from build123d import *

# Parameters (mm, degrees)
SKETCH3_R          = 4.141637382
CUT_EXTRUDE1_DEPTH = 7
FILLET2_R          = 1
FILLET3_R          = 1


with BuildPart() as part:
    # Sketch2 → Revolve1 (revolve)
    with BuildSketch(Plane.XY, mode=Mode.PRIVATE) as revolve1_sk:
        with BuildLine():
            Line((1.5, 1.5), (1.5, 3.5))
            ThreePointArc((1.5, 3.5), (1.207106781, 4.207106781), (0.5, 4.5))
            Line((0.5, 4.5), (-9.5, 4.5))
            Line((-9.5, 4.5), (-9.5, 11.5))
            Line((-9.5, 11.5), (9, 11.5))
            Line((9, 11.5), (9, 1.5))
            Line((9, 1.5), (1.5, 1.5))
        make_face()
    revolve(revolve1_sk.sketch.rotate(Axis((9, 1.5, 0), (0, 1, 0)), 270), axis=Axis((9, 1.5, 0), (0, 1, 0)))

    # Sketch3 → Cut-Extrude1 (cut)
    with BuildSketch(Plane.XZ.offset(-1.5)):
        with Locations((9, 0)):
            Circle(SKETCH3_R)
    extrude(amount=-CUT_EXTRUDE1_DEPTH, mode=Mode.SUBTRACT)

    # Fillet2
    fillet2_edges = [part.edges().sort_by_distance(p)[0] for p in [
        (9, 4.5, 18.5),
        (9, 11.5, 18.5),
    ]]
    fillet(fillet2_edges, radius=FILLET2_R)

    # Fillet3
    fillet3_edges = [part.edges().sort_by_distance(p)[0] for p in [
        (9, 1.5, 7.5),
    ]]
    fillet(fillet3_edges, radius=FILLET3_R)


solid = part.part
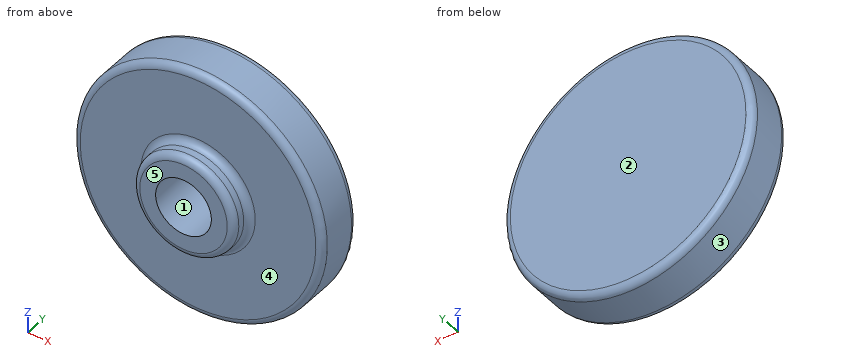
For this review, take the finished solid that the model builds, in its own axes (mm). Face numbers are marked on the shaded views. A direction names the side the tool comes from. Coordinates: 2 decimals unless noted, no trailing zeros. Write each loop counter-clockwise with the first axis right and the second up, starting at its lowest first coordinate (ties: lowest second). Pieces come first, ordered by that corner, then holes. Notation, with made-up numbers: (69, -37.75) -> (82, -37.75) arc R18 ccw to (82, -29.75) -> close; hole circle Ø9 at (51, -12). An arc over 180 degrees is marked (long way). Write each question's results on one line, items separated by ' | '. Start each with the question number.
1) Insertion check: pin 1 (10 mm diameter, centred on x = 16, z = 13, fed in from -Y); pin 2 (6 mm diameter, centred on x = 7, y = 8, fed in from -Z); pin 3 (6 mm diameter, centred on x = 1.5, y = 9, fed in from +Z); pin 4 (2.5 mm diameter, centred on x = 9.5, z = 1.5, fed in from -Y). Each pin has a flat end and moves straight along its axis. Give the tip position at first contact, or say it passes through.
2) Consider section B-B (x = 9). Write out the cut boundary in (y, z), plus the area to 3 significant figures.
3) Wall thickness on L1, parallel to Y at x = -4.5, z = -7; L2, parallel to Y at x = 11, z = 0.5; L3, parallel to Z at x = 6.5, y = 8: over which ranges is each line inside the solid? List them lowest first. Write a range as [from, to].
4) Consider section C-C (y = 9.75). Write out the cut boundary in (x, z), plus the area to 3 significant figures.
5) For the marked faces 4 and 5, list the 3-axis set-ups (+Z, -Z, +X, -X, +Y, -Y) from which the entire face can be reached by the end or side of a thin tool; tool diameter is ignored.
6) Consider section A-A (z = 0). Write out the cut boundary in (x, y).
7) The part is to be moulded in two halves that separate along Z. For the marked faces 1, 2 and 3, say which applies: +Z half, -Z half, draft (parallel to the pull), parting line (faces both ways), or undercut.
Geometry says:
1) pin 1: y = 4.5 | pin 2: z = -18.5 | pin 3: z = 17.94 | pin 4: y = 8.5
2) outline: (1.5, -6.5) arc R1 ccw to (2.5, -7.5) -> (3.5, -7.5) arc R1 cw to (4.5, -8.5) -> (4.5, -17.5) arc R1 ccw to (5.5, -18.5) -> (10.5, -18.5) arc R1 ccw to (11.5, -17.5) -> (11.5, 17.5) arc R1 ccw to (10.5, 18.5) -> (5.5, 18.5) arc R1 ccw to (4.5, 17.5) -> (4.5, 8.5) arc R1 cw to (3.5, 7.5) -> (2.5, 7.5) arc R1 ccw to (1.5, 6.5) -> (1.5, 4.14) -> (8.5, 4.14) -> (8.5, -4.14) -> (1.5, -4.14) -> close | area: 245 mm^2
3) L1: [4.5, 11.5] | L2: [8.5, 11.5] | L3: [-18.33, -3.3], [3.3, 18.33]
4) outline: circle Ø37 at (9, 0) | area: 1,080 mm^2
5) face 4: -Y | face 5: +Z, -Z, +X, -X, -Y
6) outline: (-9.5, 5.5) arc R1 ccw to (-8.5, 4.5) -> (0.5, 4.5) arc R1 cw to (1.5, 3.5) -> (1.5, 2.5) arc R1 ccw to (2.5, 1.5) -> (4.86, 1.5) -> (4.86, 8.5) -> (13.14, 8.5) -> (13.14, 1.5) -> (15.5, 1.5) arc R1 ccw to (16.5, 2.5) -> (16.5, 3.5) arc R1 cw to (17.5, 4.5) -> (26.5, 4.5) arc R1 ccw to (27.5, 5.5) -> (27.5, 10.5) arc R1 ccw to (26.5, 11.5) -> (-8.5, 11.5) arc R1 ccw to (-9.5, 10.5) -> close
7) face 1: undercut | face 2: draft | face 3: parting line
